Answer from the drawing. Dimensions are ordinates in mm from the lowest x, y and z of the part. Coordinates: 2 decimals unless noted, no trailing zeros. Write each loop counter-clockwise with the first axis right and the second up, starting at its lowest first coordinate (ties: lowest second). Pieces come first, ordered by that corner, then holes. Notation, with made-up numbers: (-9, 72.5) - (10, 72.5) arc R15 cw to (10, 83.5) - close; hole circle Ø3 at (20, 10). An arc over 180 degrees is marked (long way). Use one line per item in the form item = value. Start each with the question number.
Item 1: A cutting plane is placed at C-C (y = 1.75). Write down the section's boundary in (x, z).
Item 2: A cutting plane is placed at B-B (z = 23.18). Write down the section's boundary in (x, y).
Item 3: A cutting plane is placed at A-A (x = 20). Write down the section's boundary in (y, z), then the cut area to 3 significant figures.
Item 4: Consider probe 1 along Z at (x, y) = (20, 1.2); probe 2 along X at (y, z) = (1.25, 6.5); probe 3 along X at (y, z) = (1.9, 31). Determine where each line is inside the solid, lowest interval first.
Item 5: A cutting plane is placed at D-D (x = 52.5). Write down the section's boundary in (y, z).
Item 6: Given pin 1 (1.6 mm diameter, centred on y = 1, z = 1.5, fed in from +X); pin 2 (1 mm diameter, centred on x = 61, y = 1.5, fed in from +Z); pin 3 (10 mm diameter, centred on x = 18.5, z = 22.5, fed in from -Y); pin 4 (1 mm diameter, centred on y = 1.5, z = 1, fed in from -X), each flat-ended and moving along its own axis, determine where each tip first touches the part or whether it passes through.
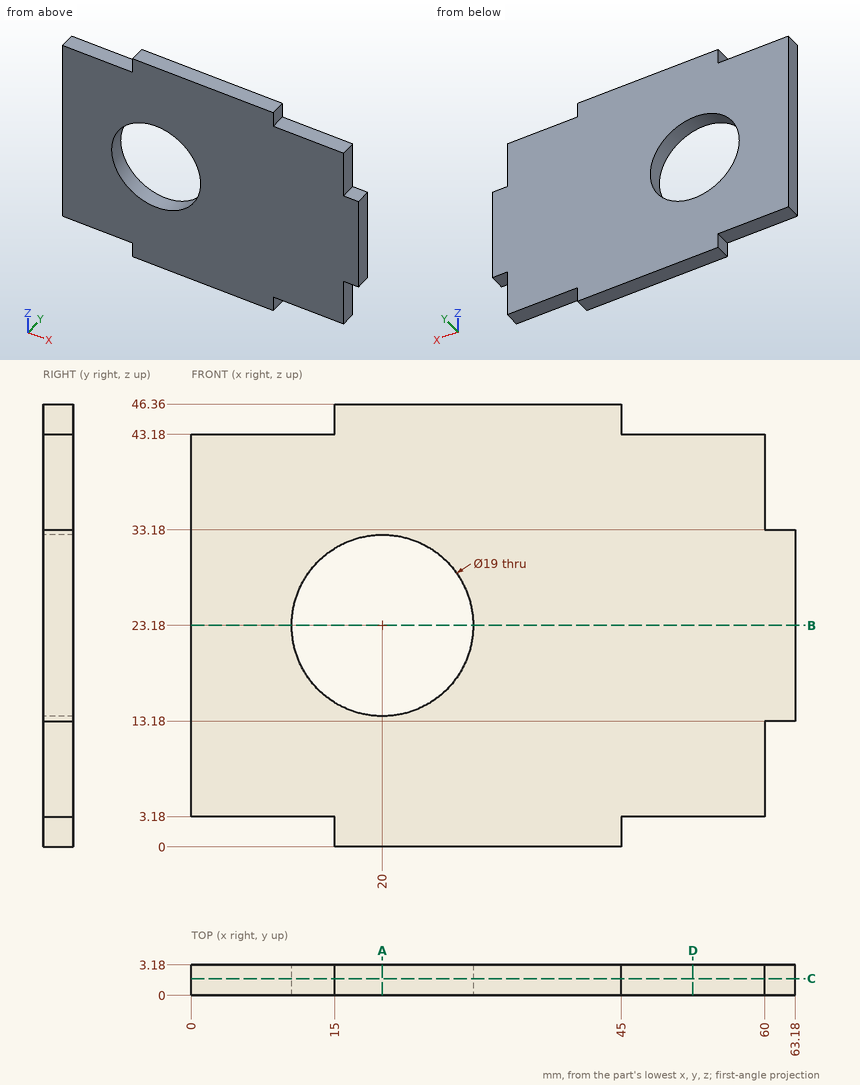
Answer:
q1.outline = (0, 3.18) - (15, 3.18) - (15, 0) - (45, 0) - (45, 3.18) - (60, 3.18) - (60, 13.18) - (63.18, 13.18) - (63.18, 33.18) - (60, 33.18) - (60, 43.18) - (45, 43.18) - (45, 46.36) - (15, 46.36) - (15, 43.18) - (0, 43.18) - close; hole circle Ø19 at (20, 23.18)
q2.outline = (0, 0) - (10.5, 0) - (10.5, 3.18) - (0, 3.18) - close; (29.5, 0) - (63.18, 0) - (63.18, 3.18) - (29.5, 3.18) - close
q3.outline = (0, 0) - (3.18, 0) - (3.18, 13.68) - (0, 13.68) - close; (0, 32.68) - (3.18, 32.68) - (3.18, 46.36) - (0, 46.36) - close
q3.area = 87.0 mm²
q4.probe_1 = 0 to 13.68, 32.68 to 46.36
q4.probe_2 = 0 to 60
q4.probe_3 = 0 to 14.61, 25.39 to 63.18
q5.outline = (0, 3.18) - (3.18, 3.18) - (3.18, 43.18) - (0, 43.18) - close
q6.pin_1 = 45
q6.pin_2 = 33.18
q6.pin_3 = through
q6.pin_4 = 15
